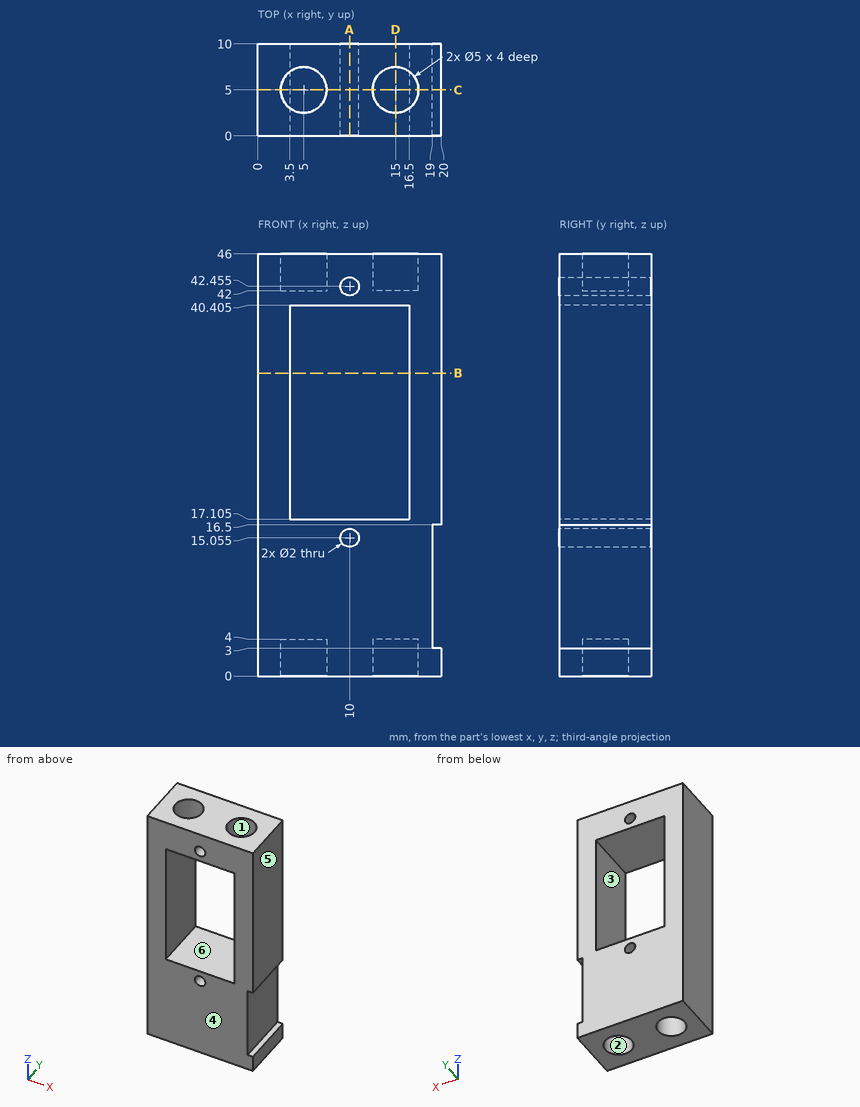
Could you check a few things on this drawing? It's one solid part, dimensions in mm from its lowest x, y, z. A direction names the side the tool comes from. Give positions to 0.01 mm unless a question says otherwise; leave off trailing zeros. Write each loop counter-clockwise with the first axis right and the second up, starting at its lowest first coordinate (ties: lowest second). Pieces come first, ordered by that corner, then holes. Notation, with made-up numbers: (-8.5, -11) - (46.5, -11) arc R29 ccw to (46.5, 11) - close; hole circle Ø8 at (-9, 44.25). An arc over 180 degrees is marked (long way). Use CSV: the item, a comma, the result in double quotes. Start each with the question number.
Item 1: For the marked faces 1, 2 and 3, which set-ups out of +Z, -Z, +X, -X, +Y, -Y let a thin tool reach every point of the face, with its end or its side?
Item 2: If we mould it in two halves opening along X, with no side actions, what happens to the marked faces 4, 5 and 6? For each: pulls with the +X half, pulls with the -X half, needs draft (parallel to the pull), parting line crosses it, or undercut.
Item 3: I want a section at A-A, the plane x = 10. Please give me the cut outline in (y, z) (3 decimals).
Item 4: I want a section at B-B, the plane z = 33. Please give me the cut outline in (x, y), then the cut area to 3 significant figures.
Item 5: I want a section at C-C, the plane y = 5. Give the number of separate pieces and of enclosed holes in the cut face, then the cut area to 3 significant figures.
Item 6: I want a section at D-D, the plane x = 15. Please give me the cut outline in (y, z) (3 decimals), then the cut area to 3 significant figures.
Item 7: I'm going to push flat-ended pins straight in: pin 1 (5.5 mm diameter, centred on x = 15, y = 5, fed in from -Z); pin 2 (1.5 mm diameter, centred on x = 4, y = 4.5, fed in from +Z). Where does each tip first touch, or does it pass through?
Item 8: If I drill on line 1 along Z through (x, y) = (16.25, 2.25) (3 decimals); line 2 along X through (y, z) = (4.25, 34); line 3 along Z through (x, y) = (4, 4.5) (3 decimals), over which ranges is the centre line in solid material (lowest first)?
Findings:
1,face 1,"+Z"
1,face 2,"-Z"
1,face 3,"+Y, -Y"
2,face 4,"needs draft"
2,face 5,"pulls with the +X half"
2,face 6,"undercut"
3,outline,"(0, 0) - (10, 0) - (10, 14.055) - (0, 14.055) - close; (0, 16.055) - (10, 16.055) - (10, 17.105) - (0, 17.105) - close; (0, 40.405) - (10, 40.405) - (10, 41.455) - (0, 41.455) - close; (0, 43.455) - (10, 43.455) - (10, 46) - (0, 46) - close"
4,outline,"(0, 0) - (3.5, 0) - (3.5, 10) - (0, 10) - close; (16.5, 0) - (20, 0) - (20, 10) - (16.5, 10) - close"
4,area,"70.0 mm2"
5,separate pieces,"1"
5,enclosed holes,"3"
5,area,"517 mm2"
6,outline,"(0, 0) - (2.5, 0) - (2.5, 4) - (7.5, 4) - (7.5, 0) - (10, 0) - (10, 17.105) - (0, 17.105) - close; (0, 40.405) - (10, 40.405) - (10, 46) - (7.5, 46) - (7.5, 42) - (2.5, 42) - (2.5, 46) - (0, 46) - close"
6,area,"187 mm2"
7,pin 1,"stops at z = 0"
7,pin 2,"stops at z = 42"
8,line 1,"z = 0 to 17.105, 40.405 to 46"
8,line 2,"x = 0 to 3.5, 16.5 to 20"
8,line 3,"z = 4 to 17.105, 40.405 to 42"
